Build history of the part. All positions in model axes, mm. Give positions to 0.01 mm unless a question says otherwise; leave off trailing zeros. Order: outer loops, then holes, each group sorted by start corner. A loop starts at its lowest first (then second) coordinate and runs counter-clockwise, first axis right, second up. Notation, with made-up numbers: (-22.75, -11) - (-2.75, -11) arc R6 ccw to (-2.75, -2) - close; hole circle Ø6 at (22.25, 35.25). An arc over 180 degrees is marked (long way). One line per item, written item: value.
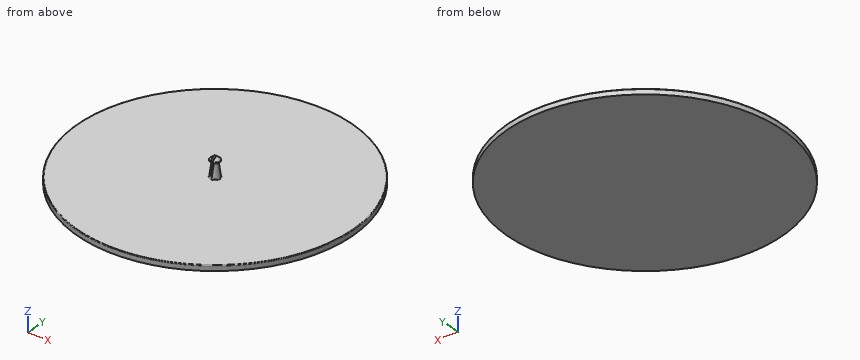
```python
from build123d import *

# Parameters (mm, degrees)
F3_DEPTH      = 1000.001
F3_DEPTH_BACK = 1000.001
F4_T4_ANGLE   = 180
F4_T9_ANGLE   = 180
F4_T12_ANGLE  = 175.5397265939
F4_T14_ANGLE  = 175.5397265939
F4_T16_ANGLE  = 194.3823817652
F4_T18_ANGLE  = 194.3823817652


# Not quite as in the source:
# - a fillet or chamfer that OpenCascade refuses, or shapes differently, is made with other operations: its cross-section is extruded or revolved along the edge and cut away or added


with BuildPart() as f1:
    # F0 (on Front) → F1 (revolve)
    with BuildSketch(Plane.XZ):
        Polygon((0, 150), (0, 0), (35, 0), (20.1401172379, 107.9545454545), (35, 110), (35, 120), align=None)
        Polygon((35, 0), (0, 0), (0, -39.4391342998), (1000, -39.4391342998), (1000, 0), align=None)
    revolve(axis=Axis((0, 0, 75), (0, 0, -1)))

    # F2 (on Front) → F3 (cut, two sides)
    with BuildSketch(Plane.XZ) as f3_sk:
        Polygon((-9.2637268826, 157.2448909283), (0, 0), (9.2637268826, 157.2448909283), (0, 157.7906424325), align=None)
    extrude(amount=F3_DEPTH, mode=Mode.SUBTRACT)
    extrude(f3_sk.sketch, amount=-F3_DEPTH_BACK, mode=Mode.SUBTRACT)

    # F4: fillet of radius 5 on 7 edges, made by hand


with BuildPart() as f4_tool2:
    # F4_s3 → F4_t4 (revolve)
    with BuildSketch(Plane.YZ):
        with BuildLine():
            ThreePointArc((39.3588989435, 0), (36.0732552402, 1.2311081928), (34.4056046895, 4.3181818182))
            Line((34.4056046895, 4.3181818182), (35, 0))
            Line((35, 0), (39.3588989435, 0))
        make_face()
    revolve(axis=Axis((0, 0, 0), (0, 0, -1)), revolution_arc=F4_T4_ANGLE)

    split(bisect_by=Plane(origin=(0, 0, 0), x_dir=(0, 1, 0), z_dir=(0.9982691489, 0, -0.0588107677)), keep=Keep.TOP)


with BuildPart() as f1_1:
    add(f1.part)

    # F4_t1: union F4_tool2
    add(f4_tool2.part)


with BuildPart() as f4_tool7:
    # F4_s8 → F4_t9 (revolve)
    with BuildSketch(Plane.YZ):
        with BuildLine():
            ThreePointArc((-39.3588989435, 0), (-36.0732552402, 1.2311081928), (-34.4056046895, 4.3181818182))
            Line((-34.4056046895, 4.3181818182), (-35, 0))
            Line((-35, 0), (-39.3588989435, 0))
        make_face()
    revolve(axis=Axis((0, 0, 0), (0, 0, -1)), revolution_arc=F4_T9_ANGLE)

    split(bisect_by=Plane(origin=(0, 0, 0), x_dir=(0, 1, 0), z_dir=(-0.9982691489, 0, -0.0588107677)), keep=Keep.TOP)


with BuildPart() as f1_2:
    add(f1_1.part)

    # F4_t6: union F4_tool7
    add(f4_tool7.part)

    # F4_s11 → F4_t12 (revolve, cut)
    with BuildSketch(Plane(origin=(0, 0, 0), x_dir=(0, 0, 1), z_dir=(-0.9992425868, 0.0389134008, 0))):
        with BuildLine():
            ThreePointArc((121.4966083995, 33.2539568673), (119.7896094353, 34.5425644925), (117.7003253876, 35))
            Line((117.7003253876, 35), (120, 35))
            Line((120, 35), (121.4966083995, 33.2539568673))
        make_face()
    revolve(axis=Axis((0, 0, 120), (0, 0, -1)), revolution_arc=F4_T12_ANGLE, mode=Mode.SUBTRACT)

    # F4_s13 → F4_t14 (revolve, cut)
    with BuildSketch(Plane(origin=(0, 0, 0), x_dir=(0, 0, 1), z_dir=(0.9992425868, -0.0389134008, 0))):
        with BuildLine():
            ThreePointArc((117.7003253876, 35), (119.7896094353, 34.5425644925), (121.4966083995, 33.2539568673))
            Line((121.4966083995, 33.2539568673), (120, 35))
            Line((120, 35), (117.7003253876, 35))
        make_face()
    revolve(axis=Axis((0, 0, 120), (0, 0, -1)), revolution_arc=F4_T14_ANGLE, mode=Mode.SUBTRACT)

    # F4_s15 → F4_t16 (revolve, cut)
    with BuildSketch(Plane(origin=(0, 0, 0), x_dir=(0, 0, 1), z_dir=(0.9921339593, 0.1251806963, 0))):
        with BuildLine():
            ThreePointArc((109.4056046895, 30.6818181818), (111.0732552402, 33.7688918072), (114.3588989435, 35))
            Line((114.3588989435, 35), (110, 35))
            Line((110, 35), (109.4056046895, 30.6818181818))
        make_face()
    revolve(axis=Axis((0, 0, 110), (0, 0, -1)), revolution_arc=F4_T16_ANGLE, mode=Mode.SUBTRACT)

    # F4_s17 → F4_t18 (revolve, cut)
    with BuildSketch(Plane(origin=(0, 0, 0), x_dir=(0, 0, 1), z_dir=(-0.9921339593, -0.1251806963, 0))):
        with BuildLine():
            ThreePointArc((114.3588989435, 35), (111.0732552402, 33.7688918072), (109.4056046895, 30.6818181818))
            Line((109.4056046895, 30.6818181818), (110, 35))
            Line((110, 35), (114.3588989435, 35))
        make_face()
    revolve(axis=Axis((0, 0, 110), (0, 0, -1)), revolution_arc=F4_T18_ANGLE, mode=Mode.SUBTRACT)

    # F4_s19 → F4_t20 (revolve, cut)
    with BuildSketch(Plane.XZ):
        with BuildLine():
            ThreePointArc((1000, -5), (998.5355339059, -1.4644660941), (995, 0))
            Line((995, 0), (1000, 0))
            Line((1000, 0), (1000, -5))
        make_face()
    revolve(axis=Axis((0, 0, 0), (0, 0, -1)), mode=Mode.SUBTRACT)


solid = f1_2.part
```
(1) Slice it at A-A, the plane z = 69. Give the cut face in (x, y), and give its area (3 significant figures).
Completed:
outline: (-4.06, -25.18) - (-4.06, 25.18) arc R25.5 ccw to start; (4.06, -25.18) arc R25.5 ccw to (4.06, 25.18) - close
area: 1,630 mm²
(2) Pin check, flat tips, straight feed: P1, Ø12, axis at x = -694.5, y = -245.5, coming from the +Z side; P2, Ø8, axis at x = -17.5, z = -3, coming from the -Y side. Stop position of each tip, or through.
Completed:
P1: z = 0
P2: y = -999.9
(3) Drill centre lines: line 1 (Z direction, x = 430.5, y = 809); line 2 (X direction, y = 24, z = 113.5); line 3 (Y direction, x = 692, z = -13.5). Where is each one in solid material? Low to high.
Completed:
line 1: -39.44 to 0
line 2: -25.37 to -6.69, 6.69 to 25.37
line 3: -721.9 to 721.9
